```python
from build123d import *

# Parameters (mm, degrees)
BOSS_EXTRUDE7_DEPTH                            = 17
BOSS_EXTRUDE7_DEPTH_BACK                       = 17
SKETCH1_R                                      = 1.45
SKETCH34_W                                     = 28.4
SKETCH34_H                                     = 7.5
CUT_EXTRUDE11_DEPTH                            = 37.521397837
SKETCH35_R                                     = 5
CUT_EXTRUDE12_DEPTH                            = 25.542055741
CSK_FOR_M3_HEX_SOCKET_COUNTERSUNK_CA_2_COUNT   = 2
CSK_FOR_M3_HEX_SOCKET_COUNTERSUNK_CA_2_PITCH   = 16.5
CSK_FOR_M3_HEX_SOCKET_COUNTERSUNK_CA_3_COUNT   = 2
CSK_FOR_M3_HEX_SOCKET_COUNTERSUNK_CA_3_PITCH   = 18
CSK_FOR_M3_HEX_SOCKET_COUNTERSUNK_CA_4_COUNT   = 2
CSK_FOR_M3_HEX_SOCKET_COUNTERSUNK_CA_4_PITCH   = 24.418230894
FILLET5_R                                      = 1
SKETCH41_W                                     = 28.5
SKETCH41_H                                     = 0.4
CUT_EXTRUDE13_DEPTH                            = 40.895175147
SKETCH47_W                                     = 24
SKETCH47_H                                     = 28
BOSS_EXTRUDE8_DEPTH                            = 3
CSK_FOR_M3_HEX_SOCKET_COUNTERSUNK_CA_5_A_COUNT = 2
CSK_FOR_M3_HEX_SOCKET_COUNTERSUNK_CA_5_A_PITCH = 9.899494937
CSK_FOR_M3_HEX_SOCKET_COUNTERSUNK_CA_6_COUNT   = 2
CSK_FOR_M3_HEX_SOCKET_COUNTERSUNK_CA_6_PITCH   = 9.899494937
CSK_FOR_M3_HEX_SOCKET_COUNTERSUNK_CA_7_COUNT   = 2
CSK_FOR_M3_HEX_SOCKET_COUNTERSUNK_CA_7_PITCH   = 9.899494937
CSK_FOR_M3_HEX_SOCKET_COUNTERSUNK_CA_8_COUNT   = 2
CSK_FOR_M3_HEX_SOCKET_COUNTERSUNK_CA_8_PITCH   = 9.899494937
SKETCH51_W                                     = 8.04998649
SKETCH51_H                                     = 7.642392238
BOSS_EXTRUDE9_DEPTH                            = 3
SKETCH53_W                                     = 29
SKETCH53_H                                     = 7.1
CUT_EXTRUDE14_DEPTH                            = 37.521397837
SKETCH54_W                                     = 16.7
SKETCH54_H                                     = 5.548131356
CUT_EXTRUDE15_DEPTH                            = 40.895175147


with BuildPart() as part:
    # Sketch1 → Boss-Extrude7 (new, two sides: drawn at the far end of the back side and taken through both)
    # profile 1 of 3: a face of its own
    with BuildSketch(Plane.XY.offset(-BOSS_EXTRUDE7_DEPTH_BACK)):
        Polygon((-14.25, 15.25), (-14.25, 11.25), (-8.25, 11.25), (-8.25, 12.25), (8.25, 12.25), (8.25, 11.25), (14.25, 11.25), (14.25, 15.25), align=None)
    # profile 2 of 3: a face of its own
    with BuildSketch(Plane.XY.offset(-BOSS_EXTRUDE7_DEPTH_BACK)):
        with BuildLine():
            Line((14.25, 4.75), (14.25, 11.25))
            Line((14.25, 11.25), (8.25, 11.25))
            Line((8.25, 11.25), (8.25, 8.011710179))
            ThreePointArc((8.25, 8.011710179), (9.502581542, 6.476954843), (10.473180033, 4.75))
            Line((10.473180033, 4.75), (14.25, 4.75))
        make_face()
        with Locations((11, 8)):
            Circle(SKETCH1_R, mode=Mode.SUBTRACT)
    # profile 3 of 3: a face of its own
    with BuildSketch(Plane.XY.offset(-BOSS_EXTRUDE7_DEPTH_BACK)):
        with BuildLine():
            Line((-8.25, 11.25), (-14.25, 11.25))
            Line((-14.25, 11.25), (-14.25, 4.75))
            Line((-14.25, 4.75), (-10.473180033, 4.75))
            ThreePointArc((-10.473180033, 4.75), (-9.502581542, 6.476954843), (-8.25, 8.011710179))
            Line((-8.25, 8.011710179), (-8.25, 11.25))
        make_face()
        with Locations((-11, 8)):
            Circle(SKETCH1_R, mode=Mode.SUBTRACT)
    extrude(amount=BOSS_EXTRUDE7_DEPTH + BOSS_EXTRUDE7_DEPTH_BACK)

    # Sketch34 → Cut-Extrude11 (cut, through all)
    with BuildSketch(Plane.ZY.offset(14.25)):
        with Locations((0, 8.5)):
            Rectangle(SKETCH34_W, SKETCH34_H)
    extrude(amount=-CUT_EXTRUDE11_DEPTH, mode=Mode.SUBTRACT)

    # Sketch35 → Cut-Extrude12 (cut, through all)
    with BuildSketch(Plane(origin=(0, 15.25, 0), x_dir=(1, 0, 0), z_dir=(0, 1, 0))):
        with Locations(Location((0, 0, 0), (0, 0, 270))):
            Circle(SKETCH35_R)
    extrude(amount=-CUT_EXTRUDE12_DEPTH, mode=Mode.SUBTRACT)

    # Sketch40 → CSK for M3 Hex Socket Countersunk Cap Sc (revolve, cut)
    with BuildSketch(Plane(origin=(-8.25, 12.25, 9), x_dir=(0, 0, -1), z_dir=(1, 0, 0))):
        Polygon((0, 0), (0, 3), (1.7, 3), (1.7, 1.66), (3.36, 0), align=None)
    csk_for_m3_hex_socket_countersunk_cap_sc = revolve(axis=Axis((-8.25, 5.9, 9), (0, 1, 0)), mode=Mode.SUBTRACT)

    # CSK for M3 Hex Socket Countersunk Ca 2: CSK for M3 Hex Socket Countersunk Cap Sc ×2
    with Locations(*[(i * CSK_FOR_M3_HEX_SOCKET_COUNTERSUNK_CA_2_PITCH, 0, 0) for i in range(1, CSK_FOR_M3_HEX_SOCKET_COUNTERSUNK_CA_2_COUNT)]):
        add(csk_for_m3_hex_socket_countersunk_cap_sc, mode=Mode.SUBTRACT)

    # CSK for M3 Hex Socket Countersunk Ca 3: CSK for M3 Hex Socket Countersunk Cap Sc ×2
    with Locations(*[(0, 0, -i * CSK_FOR_M3_HEX_SOCKET_COUNTERSUNK_CA_3_PITCH) for i in range(1, CSK_FOR_M3_HEX_SOCKET_COUNTERSUNK_CA_3_COUNT)]):
        add(csk_for_m3_hex_socket_countersunk_cap_sc, mode=Mode.SUBTRACT)

    # CSK for M3 Hex Socket Countersunk Ca 4: CSK for M3 Hex Socket Countersunk Cap Sc ×2
    with Locations(*[Vector(0.6757246285173466, 0, -0.7371541402007413) * (i * CSK_FOR_M3_HEX_SOCKET_COUNTERSUNK_CA_4_PITCH) for i in range(1, CSK_FOR_M3_HEX_SOCKET_COUNTERSUNK_CA_4_COUNT)]):
        add(csk_for_m3_hex_socket_countersunk_cap_sc, mode=Mode.SUBTRACT)

    # Fillet5
    fillet5_edges = [part.edges().sort_by_distance(p)[0] for p in [
        (-14.25, 15.25, 0),
        (14.25, 15.25, 0),
        (0, 15.25, -17),
        (0, 15.25, 17),
    ]]
    fillet(fillet5_edges, radius=FILLET5_R)

    # Sketch41 → Cut-Extrude13 (cut, through all)
    with BuildSketch(Plane.XY.offset(17)):
        with Locations((0, 4.95)):
            Rectangle(SKETCH41_W, SKETCH41_H)
    extrude(amount=-CUT_EXTRUDE13_DEPTH, mode=Mode.SUBTRACT)

    # Sketch47 → Boss-Extrude8 (add)
    with BuildSketch(Plane(origin=(0, 15.25, 0), x_dir=(1, 0, 0), z_dir=(0, 1, 0))):
        Rectangle(SKETCH47_W, SKETCH47_H)
    extrude(amount=-BOSS_EXTRUDE8_DEPTH)

    # Sketch50 → CSK for M3 Hex Socket Countersunk Ca 5 (revolve, cut)
    with BuildSketch(Plane(origin=(0, 12.25, 0), x_dir=(0, 0, -1), z_dir=(1, 0, 0))):
        Polygon((0, 0), (0, 3), (1.7, 3), (1.7, 1.66), (3.36, 0), align=None)
    csk_for_m3_hex_socket_countersunk_ca_5 = revolve(axis=Axis((0, 5.9, 0), (0, 1, 0)), mode=Mode.SUBTRACT)

    # CSK for M3 Hex Socket Countersunk Ca 5 a: CSK for M3 Hex Socket Countersunk Ca 5 ×2
    with Locations(*[Vector(-0.7071067811865477, 0, 0.7071067811865474) * (i * CSK_FOR_M3_HEX_SOCKET_COUNTERSUNK_CA_5_A_PITCH) for i in range(1, CSK_FOR_M3_HEX_SOCKET_COUNTERSUNK_CA_5_A_COUNT)]):
        add(csk_for_m3_hex_socket_countersunk_ca_5, mode=Mode.SUBTRACT)

    # CSK for M3 Hex Socket Countersunk Ca 6: CSK for M3 Hex Socket Countersunk Ca 5 ×2
    with Locations(*[Vector(-0.70710678118654, 0, -0.707106781186555) * (i * CSK_FOR_M3_HEX_SOCKET_COUNTERSUNK_CA_6_PITCH) for i in range(1, CSK_FOR_M3_HEX_SOCKET_COUNTERSUNK_CA_6_COUNT)]):
        add(csk_for_m3_hex_socket_countersunk_ca_5, mode=Mode.SUBTRACT)

    # CSK for M3 Hex Socket Countersunk Ca 7: CSK for M3 Hex Socket Countersunk Ca 5 ×2
    with Locations(*[Vector(0.7071067811865548, 0, -0.7071067811865404) * (i * CSK_FOR_M3_HEX_SOCKET_COUNTERSUNK_CA_7_PITCH) for i in range(1, CSK_FOR_M3_HEX_SOCKET_COUNTERSUNK_CA_7_COUNT)]):
        add(csk_for_m3_hex_socket_countersunk_ca_5, mode=Mode.SUBTRACT)

    # CSK for M3 Hex Socket Countersunk Ca 8: CSK for M3 Hex Socket Countersunk Ca 5 ×2
    with Locations(*[Vector(0.7071067811865477, 0, 0.7071067811865474) * (i * CSK_FOR_M3_HEX_SOCKET_COUNTERSUNK_CA_8_PITCH) for i in range(1, CSK_FOR_M3_HEX_SOCKET_COUNTERSUNK_CA_8_COUNT)]):
        add(csk_for_m3_hex_socket_countersunk_ca_5, mode=Mode.SUBTRACT)

    # Sketch51 → Boss-Extrude9 (add)
    with BuildSketch(Plane.XZ.offset(-12.25)):
        Rectangle(SKETCH51_W, SKETCH51_H)
    extrude(amount=-BOSS_EXTRUDE9_DEPTH)

    # Sketch53 → Cut-Extrude14 (cut, through all)
    with BuildSketch(Plane.ZY.offset(14.25)):
        with Locations((0, 8.7)):
            Rectangle(SKETCH53_W, SKETCH53_H)
    extrude(amount=-CUT_EXTRUDE14_DEPTH, mode=Mode.SUBTRACT)

    # Sketch54 → Cut-Extrude15 (cut, through all)
    with BuildSketch(Plane.XY.offset(17)):
        with Locations((0, 9.475934322)):
            Rectangle(SKETCH54_W, SKETCH54_H)
    extrude(amount=-CUT_EXTRUDE15_DEPTH, mode=Mode.SUBTRACT)


solid = part.part
```
The model under review builds one solid part; all positions refer to its coordinate system, in mm. A direction names the side the tool comes from. Round coordinates to 2 decimals unless told otherwise and drop trailing zeros. Loops run counter-clockwise (first coordinate to the right, second up) from the corner with the lowest first, then second, coordinate; pieces in that order, holes last. Notation, with made-up numbers: (57.5, 49) - (97.5, 49) arc R17 cw to (97.5, 77) - close; hole circle Ø8 at (73.5, 59). An arc over 180 degrees is marked (long way). Write each question's results on one line, items separated by ' | '. Start each with the question number.
Q1. Draft analysis for pull direction X (two halves, no side actions). For faces 1 (the cylindrical face through (-7.51, 14.57, 5.38)), 2 (the flat face through (-12, 5.15, 16)), state which applies: pulls with the +X half, pulls with the -X half, needs draft (parallel to the pull), parting line crosses it, or undercut.
Q2. Tool access review of faces 3 (the cylindrical face through (9.404, 6.619, 15.733)), 4 (the flat face through (12, 5.15, 16)): name each direction out of +Z, -Z, +X, -X, +Y, -Y from which nothing blocks a thin tool from reaching the whole face with its end or side.
Q3. Wall thickness on line 1 along Z through (x, y) = (-7, 14.3); line 2 along X through (y, z) = (8, -15.2); line 3 along Z through (x, y) = (11.5, 9.5): over which ranges is each line inside the solid? List them lowest first. Write a range as [from, to].
Q4. Insertion check: P1, Ø2.5, axis at x = 7, z = 7, coming from the +Y side; P2, Ø8, axis at x = -9, z = -9.5, coming from the -Y side; P3, Ø5.5, axis at x = -7, z = -7, coming from the -Y side. Each pin has a flat end and moves straight along its axis. Give the tip position at first contact, or say it passes through.
Q5. Take a section at C-C on y = 12.75. Give the boundary of the cut face in (x, z).
Q6. Take a section at B-B on x = 11. Give the boundary of the cut face in (y, z).
Q7. Take a section at A-A on z = -7. Give the boundary of the cut face in (x, y).
Q8. Take a section at D-D on x = 1.25. Give the boundary of the cut face in (y, z), plus the area to 3 significant figures.
Data:
1) face 1: undercut | face 2: needs draft
2) face 3: +Z, -Z, -Y | face 4: +Z, -Z, +X, -X, -Y
3) line 1: z = [-17, -8.7], [-5.3, 5.3], [8.7, 17] | line 2: x = [-14.25, -12.45], [-9.55, -8.35], [8.35, 9.55], [12.45, 14.25] | line 3: z = [-17, -14.5], [14.5, 17]
4) P1: passes through | P2: stops at y = 12.25 | P3: stops at y = 12.86
5) outline: (-14.25, -17) - (14.25, -17) - (14.25, 17) - (-14.25, 17) - close; hole circle Ø5.72 at (-7, -7); hole circle Ø5.72 at (-7, 7); hole circle Ø5.72 at (7, -7); hole circle Ø5.72 at (7, 7)
6) outline: (5.15, -17) - (6.55, -17) - (6.55, -14.5) - (5.15, -14.5) - close; (5.15, 14.5) - (6.55, 14.5) - (6.55, 17) - (5.15, 17) - close; (9.45, -17) - (14.25, -17) arc R1 ccw to (15.25, -16) - (15.25, 16) arc R1 ccw to (14.25, 17) - (9.45, 17) - (9.45, 14.5) - (12.25, 14.5) - (12.25, -14.5) - (9.45, -14.5) - close
7) outline: (-14.25, 12.25) - (-10.36, 12.25) - (-8.7, 13.91) - (-8.7, 15.25) - (-13.25, 15.25) arc R1 ccw to (-14.25, 14.25) - close; (-5.3, 13.91) - (-3.64, 12.25) - (3.64, 12.25) - (5.3, 13.91) - (5.3, 15.25) - (-5.3, 15.25) - close; (8.7, 13.91) - (10.36, 12.25) - (14.25, 12.25) - (14.25, 14.25) arc R1 ccw to (13.25, 15.25) - (8.7, 15.25) - close
8) outline: (12.25, -17) - (14.25, -17) arc R1 ccw to (15.25, -16) - (15.25, 16) arc R1 ccw to (14.25, 17) - (12.25, 17) - close | area: 102 mm²
